```python
from build123d import *

# Parameters (mm, degrees)
F0_W     = 58.42
F0_H     = 13.208
F0_W_2   = 1.778
F0_H_2   = 1.778
F1_DEPTH = 0.1524


with BuildPart() as f1:
    # F0 (on Front) → F1 (new body)
    with BuildSketch(Plane.XZ):
        with BuildLine():
            Line((52.490655, 5.027748), (-27.499016, 5.027748))
            ThreePointArc((-27.499016, 5.027748), (-30.939431, 3.458209), (-32.345345, -0.052249))
            Line((-32.345345, -0.052249), (-32.345345, -17.972252))
            Line((-32.345345, -17.972252), (57.570655, -17.972252))
            Line((57.570655, -17.972252), (57.570655, -0.052252))
            ThreePointArc((57.570655, -0.052252), (56.082758, 3.53985), (52.490655, 5.027748))
        make_face()
        with Locations((11.092218, -6.589826)):
            Rectangle(F0_W, F0_H, mode=Mode.SUBTRACT)
        with Locations((-27.600348, 2.790164)):
            Rectangle(F0_W_2, F0_H_2, mode=Mode.SUBTRACT)
    extrude(amount=F1_DEPTH)


solid = f1.part
```
Check sheet for the modelled part. Datum: model origin and axes. Units: mm. Round coordinates to 2 decimals unless told otherwise and drop trailing zeros. Order: outer loops, then holes, each group sorted by start corner. A loop starts at its lowest first (then second) coordinate and runs counter-clockwise, first axis right, second up. Notation, with made-up numbers: (10.25, 74.25) - (21.25, 74.25) arc R6 ccw to (21.25, 79.25) - close; hole circle Ø6 at (27, 84). An arc over 180 degrees is marked (long way). Write item = value, one per line.
Q1. Thickness scan on line 1 along X through (y, z) = (-0.1, -3.75); line 2 along Z through (x, y) = (21, -0.1); line 3 along X through (y, z) = (-0.05, 2.25). Record the ranges inside material, lowest first.
Computed:
line_1 = -32.35 to -18.12, 40.3 to 57.57
line_2 = -17.97 to -13.19, 0.01 to 5.03
line_3 = -31.79 to -28.49, -26.71 to 57.02
Q2. Section check A-A (y = -0.05). Record the boundary of the cut face in (x, z).
Computed:
outline = (-32.35, -17.97) - (57.57, -17.97) - (57.57, -0.05) arc R5.08 ccw to (52.49, 5.03) - (-27.5, 5.03) arc R5.09 ccw to (-32.35, -0.05) - close; hole (-28.49, 1.9) - (-26.71, 1.9) - (-26.71, 3.68) - (-28.49, 3.68) - close; hole (-18.12, -13.19) - (40.3, -13.19) - (40.3, 0.01) - (-18.12, 0.01) - close
Q3. Go/stop test with a flat-tipped pin: pin 1 (2 mm diameter, centred on x = 29.5, z = -13, fed in from +Y). Record where the tip stops, or that it passes through.
Computed:
pin_1 = 0
Q4. Section check C-C (x = 27). Record the boundary of the cut face in (y, z), and give its area (3 significant figures).
Computed:
outline = (-0.15, -17.97) - (0, -17.97) - (0, -13.19) - (-0.15, -13.19) - close; (-0.15, 0.01) - (0, 0.01) - (0, 5.03) - (-0.15, 5.03) - close
area = 1.49 mm^2
Q5. Section check B-B (z = -5). Record the boundary of the cut face in (x, y).
Computed:
outline = (-32.35, -0.15) - (-18.12, -0.15) - (-18.12, 0) - (-32.35, 0) - close; (40.3, -0.15) - (57.57, -0.15) - (57.57, 0) - (40.3, 0) - close
